```python
from build123d import *

# Parameters (mm, degrees)
SKETCH1_R           = 12.7
BOSS_EXTRUDE1_DEPTH = 10.16
SKETCH2_R           = 9.7
SKETCH2_R_2         = 6.175
SKETCH2_R_3         = 3.175
CUT_EXTRUDE1_DEPTH  = 7.16
FILLET1_R           = 1.75


with BuildPart() as part:
    # Sketch1 → Boss-Extrude1 (new body)
    with BuildSketch(Plane(origin=(0, 0, 0), x_dir=(1, 0, 0), z_dir=(0, 1, 0))):
        with Locations(Location((0, 0, 0), (0, 0, 270))):
            Circle(SKETCH1_R)
    extrude(amount=BOSS_EXTRUDE1_DEPTH)

    # Sketch2 → Cut-Extrude1 (cut)
    # profile 1 of 2: a face of its own
    with BuildSketch(Plane(origin=(0, 10.16, 0), x_dir=(1, 0, 0), z_dir=(0, 1, 0))):
        with Locations(Location((0, 0, 0), (0, 0, 270))):
            Circle(SKETCH2_R)
        with Locations(Location((0, 0, 0), (0, 0, 270))):
            Circle(SKETCH2_R_2, mode=Mode.SUBTRACT)
    # profile 2 of 2: a face of its own
    with BuildSketch(Plane(origin=(0, 10.16, 0), x_dir=(1, 0, 0), z_dir=(0, 1, 0))):
        with Locations(Location((0, 0, 0), (0, 0, 270))):
            Circle(SKETCH2_R_3)
    extrude(amount=-CUT_EXTRUDE1_DEPTH, mode=Mode.SUBTRACT)

    # Fillet1
    fillet1_edges = [part.edges().sort_by_distance(p)[0] for p in [
        (0, 3, -6.175),
        (0, 3, -9.7),
    ]]
    fillet(fillet1_edges, radius=FILLET1_R)


solid = part.part
```
Design review of the part built by this model. Coordinates are the model's own, in mm. A direction names the side the tool comes from. Give positions to 0.01 mm unless a question says otherwise; leave off trailing zeros. Order: outer loops, then holes, each group sorted by start corner. A loop starts at its lowest first (then second) coordinate and runs counter-clockwise, first axis right, second up. Notation, with made-up numbers: (30, 65) - (78, 65) arc R16 cw to (78, 73) - close; hole circle Ø5 at (47.25, -26.75). An arc over 180 degrees is marked (long way). Use a Markdown table: item, result. Add a question column.
(1) Add section C-C on y = 5.75. Give the boundary of the cut face in (x, z) (3 decimals).
(2) Add section B-B on z = 0. Give the boundary of the cut face in (x, y) (3 decimals), then the cut area to 3 significant figures.
(3) Add section A-A on x = 0. Give the boundary of the cut face in (y, z) (3 decimals).
(4) Machinability: for faces 1 (the face through (1.85, 7.49, 5.89)), 2 (the face through (0, 0, 0)), which of the approach directions +Z, -Z, +X, -X, +Y, -Y give a long, thin tool a straight path to every point of the face, cutting with its end or side? Answer none if there is none.
(5) Add section D-D on y = 3.5. Give the boundary of the cut face in (x, z) (3 decimals), then the cut area to 3 significant figures.
(6) Clearance check with flat-ended pins moving along their axes: P1, Ø2, axis at x = -7, y = 8.5, coming from the -Z side; P2, Ø1.9, axis at x = 1, z = -0.5, coming from the +Y side; P3, Ø3, axis at x = -9.5, y = 8.5, coming from the +Z side; P4, Ø1, axis at x = -5.5, z = 1.5, coming from the -Y side. State where each tip first meets the part, or that it passes through.
(7) Wall thickness on probe 1 along X at (y, z) = (4.75, 0) (3 decimals); probe 2 along X at (y, z) = (6, 3.25); probe 3 along X at (y, z) = (6, -2): over which ranges is each line inside the solid? List them lowest first. Write a range as [from, to].
(8) Mouldability with a two-part tool opening along X and no side actions: class faces 3 (the face through (-7.7, 5, -10.1)), 4 (the face through (-1.93, 6.63, -2.52)), 5 (the face through (-5, 10.16, -9)), 6 (the face through (2.914, 7.493, 9.252)) as +X half, -X half, draft (parallel to the pull), parting line (faces both ways), or undercut.
Report:
| question | item | result |
|---|---|---|
| 1 | outline | circle Ø25.4 at (0, 0); circle Ø12.35 at (0, 0); hole circle Ø19.4 at (0, 0); hole circle Ø6.35 at (0, 0) |
| 2 | outline | (-12.7, 0) - (12.7, 0) - (12.7, 10.16) - (9.7, 10.16) - (9.7, 4.75) arc R1.75 cw to (7.95, 3) - (7.925, 3) arc R1.75 cw to (6.175, 4.75) - (6.175, 10.16) - (3.175, 10.16) - (3.175, 3) - (-3.175, 3) - (-3.175, 10.16) - (-6.175, 10.16) - (-6.175, 4.75) arc R1.75 cw to (-7.925, 3) - (-7.95, 3) arc R1.75 cw to (-9.7, 4.75) - (-9.7, 10.16) - (-12.7, 10.16) - close |
| 2 | area | 165 mm² |
| 3 | outline | (0, -12.7) - (10.16, -12.7) - (10.16, -9.7) - (4.75, -9.7) arc R1.75 cw to (3, -7.95) - (3, -7.925) arc R1.75 cw to (4.75, -6.175) - (10.16, -6.175) - (10.16, -3.175) - (3, -3.175) - (3, 3.175) - (10.16, 3.175) - (10.16, 6.175) - (4.75, 6.175) arc R1.75 cw to (3, 7.925) - (3, 7.95) arc R1.75 cw to (4.75, 9.7) - (10.16, 9.7) - (10.16, 12.7) - (0, 12.7) - close |
| 4 | face 1 | +Y |
| 4 | face 2 | +Z, -Z, +X, -X, -Y |
| 5 | outline | circle Ø25.4 at (0, 0); circle Ø13.401 at (0, 0); hole circle Ø18.349 at (0, 0); hole circle Ø6.35 at (0, 0) |
| 5 | area | 352 mm² |
| 6 | P1 | stops at z = -11.19 |
| 6 | P2 | stops at y = 3 |
| 6 | P3 | stops at z = 9.86 |
| 6 | P4 | stops at y = 0 |
| 7 | probe 1 | x = [-12.7, -9.7], [-6.175, -3.175], [3.175, 6.175], [9.7, 12.7] |
| 7 | probe 2 | x = [-12.28, -9.14], [-5.25, 5.25], [9.14, 12.28] |
| 7 | probe 3 | x = [-12.54, -9.49], [-5.84, -2.47], [2.47, 5.84], [9.49, 12.54] |
| 8 | face 3 | parting line |
| 8 | face 4 | undercut |
| 8 | face 5 | draft |
| 8 | face 6 | undercut |
